Source: CAD feature listing. Evaluate the final solid. Frame: model axes, mm. Face numbers are marked on the shaded views. A direction names the side the tool comes from. Round coordinates to 2 decimals unless told otherwise and drop trailing zeros. Order: outer loops, then holes, each group sorted by start corner. A loop starts at its lowest first (then second) coordinate and runs counter-clockwise, first axis right, second up. Notation, with made-up numbers: (29.25, 2) - (51.25, 2) arc R21 ccw to (51.25, 13) - close; hole circle Ø10 at (53, -39). An arc over 180 degrees is marked (long way). Return JSON: item names as keys, results as strings. Group by question number.
1) Section D-D, the plane x = -8.25. Return loops of the section in (y, z) (3 decimals).
2) Contact query for flat-ended pins moving along their axis: P1, Ø8, axis at x = 4.775, y = -38.375, coming from the -Z side; P2, Ø1.6, axis at y = 28, z = 16.5, coming from the +X side (3 decimals); P3, Ø3, axis at x = 4, z = 5.5, coming from the -Y side (3 decimals). Output: stop coordinate, or through.
3) Access query for the marked faces 1, 2, 3 and 4. Directions: +Z, -Z, +X, -X, +Y, -Y. A direction counts if a zero-diameter tool reaches every point of the face in a straight line with its end or side. Return the directions, or none.
4) Mould query, pull axis Y, two halves, no side actions, for the marked faces 5, 6 and 7. Classes: pulls with the +Y half, pulls with the -Y half, needs draft (parallel to the pull), parting line crosses it, or undercut.
5) Section A-A, the plane z = 14.75. Return loops of the section in (x, y) (3 decimals), plus the area to 3 significant figures.
6) Ray query, line 1 (X direction, y = 30.5, z = 10) (3 decimals); line 2 (X direction, y = -22.5, z = 17.25) (3 decimals); line 3 (Y direction, x = 2.25, z = 15.5) (3 decimals). Return the intervals inside material, ascending. Write a range as from..to.
7) Section B-B, the plane z = 5. Return loops of the section in (x, y) (3 decimals).
8) Section C-C, the plane y = 37. Return loops of the section in (x, z) (3 decimals).
Autodesk Inventor part; units mm, degrees
ref_plane "Work Plane2" through (-11.525, -42.375, 16.25) normal (0, 0, 1) x (1, 0, 0)
ref_plane "Work Plane3" through (-12.525, -42.875, 17.75) normal (0, 0, 1) x (1, 0, 0)
ref_plane "Work Plane5" through (-12.525, -42.875, 17.75) normal (0, 0, 1) x (1, 0, 0)
ref_plane "Work Plane1" through (0, 0, 0) normal (0, 0, 1) x (1, 0, 0)
sketch "Sketch1" plane through (0, 0, 0) normal (0, 0, 1) x (1, 0, 0)
  line L0 (7.775, 18.625) -> (-4.025, 18.625)
  line L1 (-4.025, 43.875) -> (7.775, 43.875)
  line L2 (-4.025, 18.625) -> (-4.025, 43.875)
  line L3 (7.775, 23.875) -> (7.775, -22.625)
  line L4 (-4.025, 18.625) -> (6.775, 18.625)
  line L5 (6.775, 18.625) -> (6.775, 43.375)
  line L6 (6.775, 43.375) -> (-4.025, 43.375)
  line L7 (-4.025, 43.375) -> (-4.025, 18.625)
  circle A0 centre (1.775, 30.625) radius 1.3
  line L8 (7.775, -34.625) -> (2.775, -34.625)
  line L9 (2.775, -34.625) -> (2.775, -42.625)
  line L10 (7.775, -42.625) -> (2.775, -42.625)
  line L11 (5.275, -34.625) -> (-1.225, -34.625)
  line L12 (-1.225, -34.625) -> (-1.225, -42.125)
  line L13 (-1.225, -42.125) -> (5.275, -42.125)
  line L14 (5.275, -42.125) -> (5.275, -34.625)
  circle A1 centre (4.775, -38.375) radius 1.3
  line L15 (7.775, 18.625) -> (7.775, 43.875)
  line L16 (7.775, -42.625) -> (7.775, -34.625)
  point P0 (0, 0)
  point P1 (-4.025, 43.375)
  dimension "d0" = 0.5
  dimension "d1" = 1
  dimension "d30" = 0.5
  dimension "d31" = 6.5
ref_plane "Work Plane2" through (-11.525, -42.375, 16.25) normal (0, 0, 1) x (1, 0, 0)
extrude "Extrusion1" add sketch "Sketch1" along normal up to surface (16.25 mm away) contours L0 L2 L6 L5
sketch "Sketch2" plane through (-4.025, 43.375, 16.25) normal (0, 0, 1) x (1, 0, 0)
  line L0 (-7.5, -85.75) -> (-7.5, 0)
  line L1 (-7.5, 0) -> (10.8, 0)
  line L2 (10.8, -24.75) -> (10.8, 0)
  line L3 (10.8, 0) -> (10.8, -24.75)
  line L4 (0, -24.75) -> (10.8, -24.75)
  line L5 (10.8, -24.75) -> (0, -24.75)
  line L6 (0, -24.75) -> (0, -64.5)
  line L7 (0, -64.5) -> (-1.85, -64.5)
  line L8 (-1.85, -64.5) -> (-1.85, -75.5)
  line L9 (-1.85, -75.5) -> (0, -75.5)
  line L10 (-7.5, -85.75) -> (6.5, -85.75)
  line L11 (-7.5, 0.25) -> (-7.5, -85.75)
  line L12 (0, -64.75) -> (0, -75.25)
  line L13 (0, -64.75) -> (-1.6, -64.75)
  line L14 (-1.6, -75.25) -> (-1.6, -64.75)
  line L15 (0, -75.25) -> (-1.6, -75.25)
  line L16 (0, -9.75) -> (0, -20.25)
  line L17 (0, -9.75) -> (-1.6, -9.75)
  line L18 (-1.6, -20.25) -> (-1.6, -9.75)
  line L19 (0, -20.25) -> (-1.6, -20.25)
  line L20 (-1.85, -9.5) -> (0.25, -9.5)
  line L21 (0.25, -9.5) -> (0.25, -20.5)
  line L22 (0.25, -20.5) -> (-1.85, -20.5)
  line L23 (-1.85, -20.5) -> (-1.85, -9.5)
  line L24 (0, 0) -> (10.8, 0)
  line L25 (11.8, -78) -> (6.8, -78)
  line L26 (6.8, -78) -> (6.8, -86)
  line L27 (11.8, -86) -> (6.8, -86)
  line L28 (11.8, -217.75) -> (11.8, 42.25)
  line L29 (11.8, -85.75) -> (11.8, -78)
  line L30 (11.8, -78) -> (0, -78)
  line L31 (0, -78) -> (0, -75.5)
  line L32 (-7.5, -85.75) -> (11.8, -85.75)
  line L33 (0.5, -83.875) -> (0.5, -79.875)
  line L34 (0.5, -79.875) -> (2, -79.875)
  line L35 (2, -79.875) -> (2, -83.875)
  line L36 (2, -83.875) -> (0.5, -83.875)
  line L37 (0, -75.5) -> (0.25, -75.5)
  line L38 (0.25, -75.5) -> (0.25, -64.5)
  line L39 (0.25, -64.5) -> (0, -64.5)
  line L40 (2.25, -78) -> (2.25, -62.5)
  line L41 (2.25, -62.5) -> (0, -62.5)
  circle A0 centre (8.8, -81.75) radius 1.3
  line L42 (11.8, -86) -> (11.8, -78)
  point P0 (4.025, -43.375)
  point P1 (-7.5, -85.75)
  point P2 (6.5, -85.75)
  point P3 (6.8, -85.75)
  dimension "d4" = 0.25
  dimension "d5" = 0.25
  dimension "d6" = 0.25
  dimension "d7" = 0.25
  dimension "d22" = 4
  dimension "d23" = 1.875
  dimension "d24" = 1.5
  dimension "d25" = 8
  dimension "d44" = 0.25
  dimension "d45" = 2
  dimension "d46" = 2
ref_plane "Work Plane3" through (-12.525, -42.875, 17.75) normal (0, 0, 1) x (1, 0, 0)
ref_plane "Work Plane4" through (-11.525, 43.375, 17.75) normal (0, 0, 1) x (1, 0, 0)
ref_plane "Work Plane5" through (-12.525, -42.875, 17.75) normal (0, 0, 1) x (1, 0, 0)
extrude "Extrusion3" add sketch "Sketch2" along normal up to surface (1.5 mm away) contours L0 L1 L2 L4 L6 L7 L8 L9 L31 L30 L26 L32 L10 | L26 L25 L28 L32 | L30 L31 L37 L38 L39 L6 L41 L40 | A0
sketch "Sketch3" plane through (-11.525, 43.375, 17.75) normal (0, 0, 1) x (1, 0, 0)
  line L0 (18.3, 0) -> (18.3, -24.75)
  line L1 (18.3, -24.75) -> (7.5, -24.75)
  line L2 (14.3, -78) -> (14.3, -86)
  line L3 (9.75, -78) -> (19.3, -78)
  point P0 (11.525, -43.375)
  point P1 (13.3, -12.75)
  point P2 (7.5, -78)
  dimension "d13" = 5
  dimension "d14" = 12
hole "Hole1" at (1.775, 30.625, 17.75) direction (0, 0, -1) diameter 3.2 end through all counterbore diameter 6 counterbore depth 16.5
sketch "Sketch4" plane through (-4.025, 43.375, 16.25) normal (0, 0, -1) x (-1, 0, 0)
  line L0 (-2.25, -78) -> (-11.8, -78)
  line L1 (-11.8, -78) -> (-11.8, -85.75)
  line L2 (-4.8, -78) -> (-11.8, -78)
  line L3 (-11.8, -78) -> (-11.8, -85.75)
  line L4 (-11.8, -85.75) -> (-4.8, -85.75)
  line L5 (-4.8, -85.75) -> (-4.8, -78)
  point P0 (-4.025, -43.375)
  point P1 (0, -78)
  dimension "d32" = 7
ref_plane "Work Plane6" through (2.775, -42.625, 10) normal (0, 0, 1) x (1, 0, 0)
extrude "Extrusion4" add sketch "Sketch4" along normal up to surface (6.25 mm away)
sketch "Sketch5" plane through (-11.525, -42.375, 17.75) normal (0, 0, 1) x (1, 0, 0)
  line L0 (19.3, 7.75) -> (19.3, 0)
  line L1 (9.75, 7.75) -> (19.3, 7.75)
  point P0 (11.525, 42.375)
  point P1 (16.3, 4)
  point P2 (7.5, 7.75)
  dimension "d35" = 3
  dimension "d36" = 3.75
hole "Hole2" at (4.775, -38.375, 17.75) direction (0, 0, -1) diameter 3.2 end through all counterbore diameter 6 counterbore depth 2
properties part number "Display_Cover"
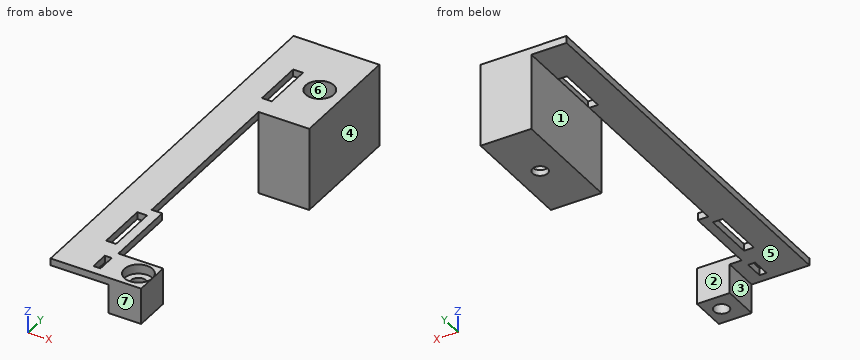
Geometry check:
{
 "1": {"outline": "(-42.375, 16.25) - (43.375, 16.25) - (43.375, 17.75) - (-42.375, 17.75) - close"},
 "2": {"P1": "z = 10", "P2": "x = 6.775", "P3": "y = 18.625"},
 "3": {"face 1": "-Z, -X, +Y, -Y", "face 2": "+Z, -Z, +X", "face 3": "-Z, -X, -Y", "face 4": "+Z, -Z, +X, +Y"},
 "4": {"face 5": "needs draft", "face 6": "undercut", "face 7": "pulls with the -Y half"},
 "5": {"outline": "(-4.025, 18.625) - (6.775, 18.625) - (6.775, 43.375) - (-4.025, 43.375) - close; (0.775, -42.375) - (7.775, -42.375) - (7.775, -34.625) - (0.775, -34.625) - close; hole circle Ø6 at (1.775, 30.625); hole circle Ø3.2 at (4.775, -38.375)", "area": "285 mm2"},
 "6": {"line 1": "-4.025..-1.222, 4.772..6.775", "line 2": "-11.525..-5.875, -3.775..-1.775", "line 3": "-42.375..-34.625, 18.625..27.663, 33.587..43.375"},
 "7": {"outline": "(-4.025, 18.625) - (6.775, 18.625) - (6.775, 43.375) - (-4.025, 43.375) - close; hole circle Ø6 at (1.775, 30.625)"},
 "8": {"outline": "(-11.525, 16.25) - (-4.025, 16.25) - (-4.025, 0) - (6.775, 0) - (6.775, 17.75) - (-11.525, 17.75) - close"}
}
